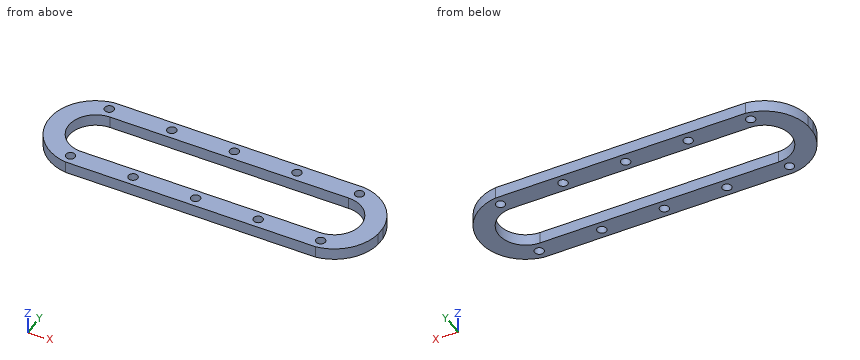
from build123d import *

# Parameters (mm, degrees)
SKETCH1_W                    = 176.276
SKETCH1_H                    = 49.149
BOSS_EXTRUDE1_DEPTH          = 6.35
CUT_EXTRUDE1_DEPTH           = 92.719875677
CUT_EXTRUDE4_DEPTH           = 92.719875677
F_10_0_1935_DIAMETER_HOLE1_D = 4.9149


with BuildPart() as part:
    # Sketch1 → Boss-Extrude1 (new body)
    with BuildSketch(Plane.XY):
        Rectangle(SKETCH1_W, SKETCH1_H)
    extrude(amount=BOSS_EXTRUDE1_DEPTH)

    # Sketch2 → Cut-Extrude1 (cut, through all)
    with BuildSketch(Plane.XY.offset(6.35)):
        with BuildLine():
            Line((63.5, -14.351), (-63.5, -14.351))
            ThreePointArc((-63.5, -14.351), (-77.851, 0), (-63.5, 14.351))
            Line((-63.5, 14.351), (63.5, 14.351))
            ThreePointArc((63.5, 14.351), (77.851, 0), (63.5, -14.351))
        make_face()
    extrude(amount=-CUT_EXTRUDE1_DEPTH, mode=Mode.SUBTRACT)

    # Sketch8 → Cut-Extrude4 (cut, through all)
    with BuildSketch(Plane.XY.offset(6.35)):
        with BuildLine():
            ThreePointArc((-88.138, 2.504831531), (-81.209963357, 17.310760321), (-66.565807357, 24.5745))
            Line((-66.565807357, 24.5745), (-88.138, 24.5745))
            Line((-88.138, 24.5745), (-88.138, 2.504831531))
        make_face()
        with BuildLine():
            ThreePointArc((-66.565807357, -24.5745), (-81.209963357, -17.310760321), (-88.138, -2.504831531))
            Line((-88.138, -2.504831531), (-88.138, -24.5745))
            Line((-88.138, -24.5745), (-66.565807357, -24.5745))
        make_face()
        with BuildLine():
            Line((88.138, 24.5745), (66.565807357, 24.5745))
            ThreePointArc((66.565807357, 24.5745), (81.209963357, 17.310760321), (88.138, 2.504831531))
            Line((88.138, 2.504831531), (88.138, 24.5745))
        make_face()
        with BuildLine():
            Line((88.138, -24.5745), (88.138, -2.504831531))
            ThreePointArc((88.138, -2.504831531), (81.209963357, -17.310760321), (66.565807357, -24.5745))
            Line((66.565807357, -24.5745), (88.138, -24.5745))
        make_face()
    extrude(amount=-CUT_EXTRUDE4_DEPTH, mode=Mode.SUBTRACT)

    # #10 (0.1935) Diameter Hole1 (through all)
    with Locations(Plane.XY.offset(6.35)):
        with Locations((-66.565807357, 19.46275), (-33.282903678, 19.46275), (0, 19.46275), (33.282903678, 19.46275), (66.565807357, 19.46275), (66.565807357, -19.46275), (33.282903678, -19.46275), (0, -19.46275), (-33.282903678, -19.46275), (-66.565807357, -19.46275)):
            Hole(F_10_0_1935_DIAMETER_HOLE1_D / 2)


solid = part.part
The listing builds one solid part. Answer for the finished solid, in the listing's coordinates (mm). Coordinates: 2 decimals unless noted, no trailing zeros. Write each loop counter-clockwise with the first axis right and the second up, starting at its lowest first coordinate (ties: lowest second). Pieces come first, ordered by that corner, then holes. Notation, with made-up numbers: (33.25, 50.25) -> (49.25, 50.25) arc R27 cw to (49.25, 80.25) -> close; hole circle Ø11 at (42, 24.25). An arc over 180 degrees is marked (long way). One line per question, with ' | ' between items.
1. Section C-C (y = 0) is taken. Determine the outline of the cut face in (x, z).
Verdict:
outline: (-88.14, 0) -> (-77.85, 0) -> (-77.85, 6.35) -> (-88.14, 6.35) -> close; (77.85, 0) -> (88.14, 0) -> (88.14, 6.35) -> (77.85, 6.35) -> close
2. Given pin 1 Ø1.5 at (y, z) = (4.5, 1) entering from -X; pin 2 Ø1 at (x, z) = (69, 2) entering from +Y (3 decimals), each flat-ended and moving along its own axis, determine where each tip first touches the part or whether it passes through.
Verdict:
pin 1: stops at x = -87.98 | pin 2: stops at y = 24.255
3. Section A-A (x = 0) is taken. Determine the outline of the cut face in (y, z), and give its area (3 significant figures).
Verdict:
outline: (-24.57, 0) -> (-21.92, 0) -> (-21.92, 6.35) -> (-24.57, 6.35) -> close; (-17.01, 0) -> (-14.35, 0) -> (-14.35, 6.35) -> (-17.01, 6.35) -> close; (14.35, 0) -> (17.01, 0) -> (17.01, 6.35) -> (14.35, 6.35) -> close; (21.92, 0) -> (24.57, 0) -> (24.57, 6.35) -> (21.92, 6.35) -> close | area: 67.4 mm^2
4. Straight lines are drawn through the part: line 1 (X direction, y = 0, z = 4.5); line 2 (Y direction, x = 11, z = 4.25); line 3 (Y direction, x = 34, z = 1.25). For each, find the intervals that lie inside material, in ascending order.
Verdict:
line 1: x = -88.14 to -77.85, 77.85 to 88.14 | line 2: y = -24.57 to -14.35, 14.35 to 24.57 | line 3: y = -24.57 to -21.81, -17.11 to -14.35, 14.35 to 17.11, 21.81 to 24.57
5. Section D-D (z = 2.5) is taken. State how many separate pieces and enclosed holes the cut face has, and give its area (3 significant figures).
Verdict:
separate pieces: 1 | enclosed holes: 11 | area: 3,680 mm^2
6. Section B-B (x = -29) is taken. Determine the outline of the cut face in (y, z), and give its area (3 significant figures).
Verdict:
outline: (-24.57, 0) -> (-14.35, 0) -> (-14.35, 6.35) -> (-24.57, 6.35) -> close; (14.35, 0) -> (24.57, 0) -> (24.57, 6.35) -> (14.35, 6.35) -> close | area: 130 mm^2
